Input: part model. Units: mm. Frame: model coordinates. A direction names the side the tool comes from. Round coordinates to 2 decimals unless told otherwise and drop trailing zeros. Loops run counter-clockwise (first coordinate to the right, second up) from the corner with the lowest first, then second, coordinate; pieces in that order, holes last.
(1) Draft query along X for faces 1 (the face through (13, -20.5, 9)), 2 (the face through (38, -3, 9)), 3 (the face through (-31, 0, 19)). Return one class per face: released by +X, released by -X, zero draft, split by the parting line, or undercut.
(2) Cut plane B-B, the plane y = -5. Output: boundary loops of the cut face in (x, z), and give its area (3 significant figures).
(3) Access query for faces 4 (the face through (20, -11, 0)), 5 (the face through (-25, -12.5, 20)), 6 (the face through (-12, -26, 2)). Directions: +Z, -Z, +X, -X, +Y, -Y. A direction counts if a zero-diameter tool reaches every point of the face in a straight line with its end or side. Return the directions, or none.
(4) Line query: line 1 (X direction, y = 3, z = 19); line 2 (Z direction, x = 1.5, y = 0.5); line 3 (Y direction, x = 27, z = 16.5). Output: solid intervals per line, ascending.
(5) Cut plane D-D, the plane y = -18. Output: boundary loops of the cut face in (x, z).
(6) First-contact query: pin 1 Ø4 at (x, y) = (31, 0) entering from -Z; pin 2 Ø6.5 at (x, z) = (-16.5, 18.5) entering from -Y; pin 3 Ø4 at (x, y) = (-26, -27) entering from -Z. Flat tips, straight axial feed; report the tip coordinate or a pass-through.
(7) Cut plane A-A, the plane x = -25. Output: boundary loops of the cut face in (y, z), and give its area (4 significant figures).
(8) Cut plane C-C, the plane z = 19.5. Give the number of separate pieces and of enclosed holes in the cut face, and give its area (3 significant figures).
from build123d import *

# Parameters (mm, degrees)
SKETCH_1_W           = 70
SKETCH_1_H           = 30
EXTRUDE_1_DEPTH      = 27
CUT_EXTRUDE_1_DEPTH  = 47.679760068
SKETCH_3_R           = 1.65
CUT_EXTRUDE_2_DEPTH  = 47.679760068
SKETCH_4_W           = 21
SKETCH_4_H           = 8.5
CUT_EXTRUDE_3_DEPTH  = 47.679760068
SKETCH_7_R           = 11.25
CUT_EXTRUDE_5_DEPTH  = 47.679760068
SKETCH_8_W           = 21.5
SKETCH_8_H           = 21.5
EXTRUDE_2_DEPTH      = 8
SKETCH_10_R          = 1.5
CUT_EXTRUDE_6_DEPTH  = 54.422841557
SKETCH_12_W          = 35
SKETCH_12_H          = 21.5
EXTRUDE_3_DEPTH      = 3
SKETCH_13_R          = 3
CUT_EXTRUDE_7_DEPTH  = 15
SKETCH_14_R          = 1.65
EXTRUDE_4_DEPTH      = 27
SKETCH_15_W          = 27
SKETCH_15_H          = 30
EXTRUDE_5_DEPTH      = 3
EXTRUDE_START        = 5.5
SKETCH_16_R          = 3
EXTRUDE_6_DEPTH      = 5.5
SKETCH_22_W          = 26
SKETCH_22_H          = 15
CUT_EXTRUDE_9_DEPTH  = 8
EXTRUDE_START_2      = 8
SKETCH_20_R          = 11.25
EXTRUDE_8_DEPTH      = 8
CUT_EXTRUDE_8_DEPTH  = 8
SKETCH_23_W          = 26
SKETCH_23_H          = 20
EXTRUDE_9_DEPTH      = 17
SKETCH_24_R          = 2
CUT_EXTRUDE_10_DEPTH = 64.837684795
SKETCH_25_R          = 3.75
CUT_EXTRUDE_11_DEPTH = 5
SKETCH_26_R          = 3.1
CUT_EXTRUDE_12_DEPTH = 16
SKETCH_27_R          = 1.25
CUT_EXTRUDE_13_DEPTH = 10
SKETCH_28_W          = 2
SKETCH_28_H          = 12.06571985
CUT_EXTRUDE_14_DEPTH = 16
FILLET_1_R           = 2
SKETCH_29_W          = 20
SKETCH_29_H          = 5
CUT_EXTRUDE_15_DEPTH = 89.945207853


with BuildPart() as part:
    # 草图1 → 凸台-拉伸1 (new body)
    with BuildSketch(Plane.XY):
        Rectangle(SKETCH_1_W, SKETCH_1_H)
    extrude(amount=EXTRUDE_1_DEPTH)

    # 草图2 → 切除-拉伸1 (cut, through all)
    with BuildSketch(Plane.XY.offset(27)):
        with BuildLine():
            Line((28.228756555, -15), (35, -15))
            Line((35, -15), (35, 0))
            ThreePointArc((35, 0), (33.228756555, -8.228756555), (28.228756555, -15))
        make_face()
        with BuildLine():
            ThreePointArc((28.228756555, 15), (33.228756555, 8.228756555), (35, 0))
            Line((35, 0), (35, 15))
            Line((35, 15), (28.228756555, 15))
        make_face()
    extrude(amount=-CUT_EXTRUDE_1_DEPTH, mode=Mode.SUBTRACT)

    # 草图3 → 切除-拉伸2 (cut, through all)
    with BuildSketch(Plane.XY.offset(27)):
        with Locations((31, 0)):
            Circle(SKETCH_3_R)
        with Locations((26.313708499, 11.313708499)):
            Circle(SKETCH_3_R)
        with Locations(Location((26.313708499, -11.313708499, 0), (0, 0, 180))):
            Circle(SKETCH_3_R)
        with Locations(Location((3.686291501, 11.313708499, 0), (0, 0, 180))):
            Circle(SKETCH_3_R)
        with Locations((3.686291501, -11.313708499)):
            Circle(SKETCH_3_R)
        with Locations((-1, 0)):
            Circle(SKETCH_3_R)
    extrude(amount=-CUT_EXTRUDE_2_DEPTH, mode=Mode.SUBTRACT)

    # 草图4 → 切除-拉伸3 (cut, through all)
    with BuildSketch(Plane.XY.offset(27)):
        with Locations((-24.5, 10.75)):
            Rectangle(SKETCH_4_W, SKETCH_4_H)
    extrude(amount=-CUT_EXTRUDE_3_DEPTH, mode=Mode.SUBTRACT)

    # 草图7 → 切除-拉伸5 (cut, through all)
    with BuildSketch(Plane(origin=(0, 0, 0), x_dir=(-1, 0, 0), z_dir=(0, 0, -1))):
        with Locations((-15, 0)):
            Circle(SKETCH_7_R)
    extrude(amount=-CUT_EXTRUDE_5_DEPTH, mode=Mode.SUBTRACT)

    # 草图8 → 凸台-拉伸2 (add)
    with BuildSketch(Plane(origin=(0, 0, 0), x_dir=(-1, 0, 0), z_dir=(0, 0, -1))):
        with Locations((24.25, -4.25)):
            Rectangle(SKETCH_8_W, SKETCH_8_H)
    extrude(amount=EXTRUDE_2_DEPTH)

    # 草图10 → 切除-拉伸6 (cut, through all)
    with BuildSketch(Plane.XZ.offset(15)):
        with Locations(Location((-17.5, 19.95, 0), (0, 0, 270))):
            Circle(SKETCH_10_R)
        with Locations(Location((-32.5, 19.95, 0), (0, 0, 270))):
            Circle(SKETCH_10_R)
    extrude(amount=-CUT_EXTRUDE_6_DEPTH, mode=Mode.SUBTRACT)

    # 草图12 → 凸台-拉伸3 (add)
    with BuildSketch(Plane.ZY.offset(35)):
        with Locations((9.5, -4.25)):
            Rectangle(SKETCH_12_W, SKETCH_12_H)
    extrude(amount=EXTRUDE_3_DEPTH)

    # 草图13 → 切除-拉伸7 (cut)
    with BuildSketch(Plane.XZ.offset(15)):
        with Locations(Location((-32.5, 19.95, 0), (0, 0, 270))):
            Circle(SKETCH_13_R)
        with Locations(Location((-17.5, 19.95, 0), (0, 0, 270))):
            Circle(SKETCH_13_R)
    extrude(amount=-CUT_EXTRUDE_7_DEPTH, mode=Mode.SUBTRACT)

    # 草图14 → 凸台-拉伸4 (add)
    with BuildSketch(Plane.XY.offset(27)):
        Polygon((28.228756555, -15), (35, -15), (35, 0), (35, 15), (28.228756555, 15), (28.228756555, 12.920752662), (28.228756555, 9.706664336), (28.228756555, 0), (28.228756555, -9.706664336), (28.228756555, -12.920752662), align=None)
        with Locations((31, 0)):
            Circle(SKETCH_14_R, mode=Mode.SUBTRACT)
    extrude(amount=-EXTRUDE_4_DEPTH)

    # 草图15 → 凸台-拉伸5 (add)
    with BuildSketch(Plane(origin=(35, 0, 0), x_dir=(0, 0, -1), z_dir=(1, 0, 0))):
        with Locations((-13.5, 0)):
            Rectangle(SKETCH_15_W, SKETCH_15_H)
    extrude(amount=EXTRUDE_5_DEPTH)

    # 草图16 → 凸台-拉伸6 (add)
    with BuildSketch(Plane.XZ.offset(15).offset(EXTRUDE_START)):
        Polygon((-13.5, 0), (38, 0), (38, 27), (-38, 27), (-38, -8), (-13.5, -8), align=None)
        with Locations(Location((-32.5, 19.95, 0), (0, 0, 270))):
            Circle(SKETCH_16_R, mode=Mode.SUBTRACT)
        with Locations(Location((-17.5, 19.95, 0), (0, 0, 270))):
            Circle(SKETCH_16_R, mode=Mode.SUBTRACT)
    extrude(amount=-EXTRUDE_6_DEPTH)

    # 草图22 → 切除-拉伸9 (cut)
    with BuildSketch(Plane.XZ.offset(20.5)):
        with Locations((-25, 19.5)):
            Rectangle(SKETCH_22_W, SKETCH_22_H)
    extrude(amount=-CUT_EXTRUDE_9_DEPTH, mode=Mode.SUBTRACT)

    # 草图20 → 凸台-拉伸8 (add)
    with BuildSketch(Plane(origin=(0, 0, 0), x_dir=(-1, 0, 0), z_dir=(0, 0, -1)).offset(EXTRUDE_START_2)):
        Polygon((14, 15), (-38, 15), (-38, -20.5), (13.5, -20.5), (13.5, 6.5), (14, 6.5), align=None)
        with Locations((-15, 0)):
            Circle(SKETCH_20_R, mode=Mode.SUBTRACT)
    extrude(amount=-EXTRUDE_8_DEPTH)

    # 草图21 → 切除-拉伸8 (cut)
    with BuildSketch(Plane(origin=(0, 0, -8), x_dir=(-1, 0, 0), z_dir=(0, 0, -1))):
        with BuildLine():
            Line((-27.816005618, -16), (-2.183994382, -16))
            ThreePointArc((-2.183994382, -16), (-15, 20.5), (-27.816005618, -16))
        make_face()
    extrude(amount=-CUT_EXTRUDE_8_DEPTH, mode=Mode.SUBTRACT)

    # 草图23 → 凸台-拉伸9 (add)
    with BuildSketch(Plane.XZ.offset(20.5)):
        with Locations((-25, 2)):
            Rectangle(SKETCH_23_W, SKETCH_23_H)
    extrude(amount=EXTRUDE_9_DEPTH)

    # 草图24 → 切除-拉伸10 (cut, through all)
    with BuildSketch(Plane(origin=(0, 0, -8), x_dir=(-1, 0, 0), z_dir=(0, 0, -1))):
        with Locations((17, -27)):
            Circle(SKETCH_24_R)
        with Locations((25, -27)):
            Circle(SKETCH_24_R)
    extrude(amount=-CUT_EXTRUDE_10_DEPTH, mode=Mode.SUBTRACT)

    # 草图25 → 切除-拉伸11 (cut)
    with BuildSketch(Plane(origin=(0, 0, -8), x_dir=(-1, 0, 0), z_dir=(0, 0, -1))):
        with Locations((17, -27)):
            Circle(SKETCH_25_R)
        with Locations((25, -27)):
            Circle(SKETCH_25_R)
    extrude(amount=-CUT_EXTRUDE_11_DEPTH, mode=Mode.SUBTRACT)

    # 草图26 → 切除-拉伸12 (cut)
    with BuildSketch(Plane.XZ.offset(37.5)):
        with Locations(Location((-31, 7, 0), (0, 0, 270))):
            Circle(SKETCH_26_R)
    extrude(amount=-CUT_EXTRUDE_12_DEPTH, mode=Mode.SUBTRACT)

    # 草图27 → 切除-拉伸13 (cut)
    with BuildSketch(Plane.XZ.offset(21.5)):
        with Locations(Location((-31, 7, 0), (0, 0, 270))):
            Circle(SKETCH_27_R)
    extrude(amount=-CUT_EXTRUDE_13_DEPTH, mode=Mode.SUBTRACT)

    # 草图28 → 切除-拉伸14 (cut)
    with BuildSketch(Plane.XZ.offset(37.5)):
        with Locations((-31, -1.967140075)):
            Rectangle(SKETCH_28_W, SKETCH_28_H)
    extrude(amount=-CUT_EXTRUDE_14_DEPTH, mode=Mode.SUBTRACT)

    # 圆角1
    fillet_1_edges = [part.edges().sort_by_distance(p)[0] for p in [
        (-32, -29.5, 4.06571985),
        (-30, -29.5, 4.06571985),
    ]]
    fillet(fillet_1_edges, radius=FILLET_1_R)

    # 草图29 → 切除-拉伸15 (cut, through all)
    with BuildSketch(Plane.ZY.offset(38)):
        with Locations((2, -35)):
            Rectangle(SKETCH_29_W, SKETCH_29_H)
    extrude(amount=-CUT_EXTRUDE_15_DEPTH, mode=Mode.SUBTRACT)


solid = part.part
Reported:
1. face 1: zero draft
1. face 2: released by +X
1. face 3: undercut
2. outline: (-38, -8) - (-4.88, -8) - (-4.88, 0) - (4.92, 0) - (4.92, 27) - (-38, 27) - close; (25.08, 0) - (34.88, 0) - (34.88, -8) - (38, -8) - (38, 27) - (25.08, 27) - close; hole circle Ø6 at (-32.5, 19.95); hole circle Ø6 at (-17.5, 19.95)
2. area: 1,740 mm2
3. face 4: -Z
3. face 5: +Z, -X, -Y
3. face 6: +Z, -Z, +X, -Y
4. line 1: x = -38 to -33.66, -31.34 to -18.66, -16.34 to 4.16, 25.84 to 38
4. line 2: z = 0 to 27
4. line 3: y = -20.5 to -12.81, -9.81 to 9.81, 12.81 to 15
5. outline: (-38, -8) - (38, -8) - (38, 27) - (-12, 27) - (-12, 12) - (-38, 12) - close; hole circle Ø2.5 at (-31, 7)
6. pin 1: stops at z = 0
6. pin 2: stops at y = -12.5
6. pin 3: stops at z = -3
7. outline: (-32.5, -8) - (-30.75, -8) - (-30.75, -3) - (-29, -3) - (-29, 12) - (-32.5, 12) - close; (-25, -3) - (-23.25, -3) - (-23.25, -8) - (6.5, -8) - (6.5, 27) - (-12.5, 27) - (-12.5, 12) - (-25, 12) - close
7. area: 967.5 mm2
8. separate pieces: 3
8. enclosed holes: 7
8. area: 1,650 mm2
